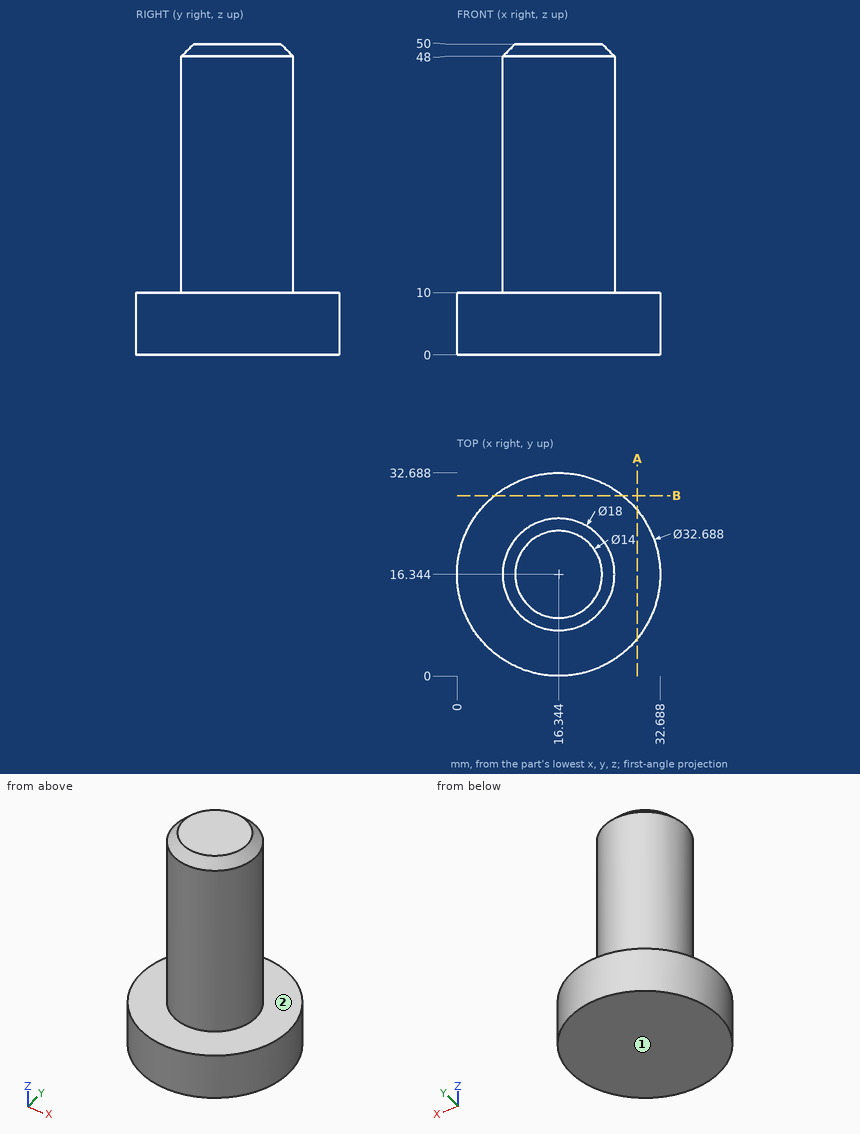
Could you check a few things on this drawing? It's one solid part, dimensions in mm from its lowest x, y, z. A direction names the side the tool comes from. Coordinates: 2 decimals unless noted, no trailing zeros. Write each loop counter-clockwise with the first axis right and the second up, starting at its lowest first coordinate (ties: lowest second). Pieces come first, ordered by that corner, then holes. Notation, with made-up numbers: (23.25, 10) - (32.25, 10) arc R31 ccw to (32.25, 42) - close; hole circle Ø2 at (-15.75, 21). An arc over 180 degrees is marked (long way). Return JSON: item names as keys, results as strings. Group by question number.
Item 1: Which directions (+Z, -Z, +X, -X, +Y, -Y) give clear straight access to the entire face, cutting with the end or side of a thin tool? Please do the marked faces 1 and 2.
Item 2: If we section it at A-A (x = 29): Write out the boundary of the cut face in (y, z).
Item 3: Please list where these lines run through material, in increasing order: probe 1 along Z at (x, y) = (7.5, 19.5); probe 2 along Y at (x, z) = (22.5, 6) (1 decimal); probe 3 along Y at (x, z) = (11, 47.5) (1 decimal).
Item 4: I'm going to push flat-ended pins straight in: pin 1 Ø1.5 at (x, z) = (11, 18.5) entering from -Y (1 decimal); pin 2 Ø4 at (y, z) = (23.5, 24) entering from -X; pin 3 Ø8 at (x, z) = (12, 43.5) entering from +Y. Where does each tip first touch, or does it pass through?
Return value:
{
 "1": {"face 1": "-Z, +X, -X, +Y, -Y", "face 2": "+Z"},
 "2": {"outline": "(6, 0) - (26.69, 0) - (26.69, 10) - (6, 10) - close"},
 "3": {"probe 1": "z = 0 to 10", "probe 2": "y = 1.2 to 31.5", "probe 3": "y = 9.1 to 23.6"},
 "4": {"pin 1": "stops at y = 8.6", "pin 2": "stops at x = 8.97", "pin 3": "stops at y = 25.34"}
}
